Read the model definition and answer for the solid it produces. Units are mm, in the model's axes. Face numbers are marked on the shaded views. A direction names the side the tool comes from. Coordinates: 2 decimals unless noted, no trailing zeros. Order: outer loops, then holes, each group sorted by start corner. A loop starts at its lowest first (then second) coordinate and runs counter-clockwise, first axis right, second up. Notation, with made-up numbers: (36.5, 26.25) - (91.5, 26.25) arc R18 cw to (91.5, 49.25) - close; hole circle Ø4 at (66, 86). An arc over 180 degrees is marked (long way). Write item = value, one per line.
from build123d import *

# Parameters (mm, degrees)
F0_W     = 10.414
F0_H     = 140.97
F1_DEPTH = 1.27
F2_W     = 10.414
F2_H     = 1.27
F3_DEPTH = 67.564
F4_DEPTH = 67.564
F6_DEPTH = 1.27
F8_DEPTH = 1.27


with BuildPart() as f1:
    # F0 (on Top) → F1 (new body)
    with BuildSketch(Plane.XY):
        Rectangle(F0_W, F0_H)
    extrude(amount=F1_DEPTH)

    # F2 (on face) → F3 (join)
    with BuildSketch(Plane.XY.offset(1.27)):
        with Locations((0, -69.85)):
            Rectangle(F2_W, F2_H)
    extrude(amount=F3_DEPTH)

    # F2 (on face) → F4 (join)
    with BuildSketch(Plane.XY.offset(1.27)):
        with Locations((0, 69.85)):
            Rectangle(F2_W, F2_H)
    extrude(amount=F4_DEPTH)

    # F5 (on face) → F6 (join)
    with BuildSketch(Plane.YZ.offset(5.207)):
        Polygon((69.215, 1.27), (-69.215, 68.834), (-69.215, 1.27), align=None)
    extrude(amount=-F6_DEPTH)

    # F7 (on face) → F8 (join)
    with BuildSketch(Plane(origin=(-5.207, 0, 0), x_dir=(0, -1, 0), z_dir=(-1, 0, 0))):
        Polygon((69.215, 1.27), (-69.215, 68.834), (-69.215, 1.27), align=None)
    extrude(amount=-F8_DEPTH)


solid = f1.part
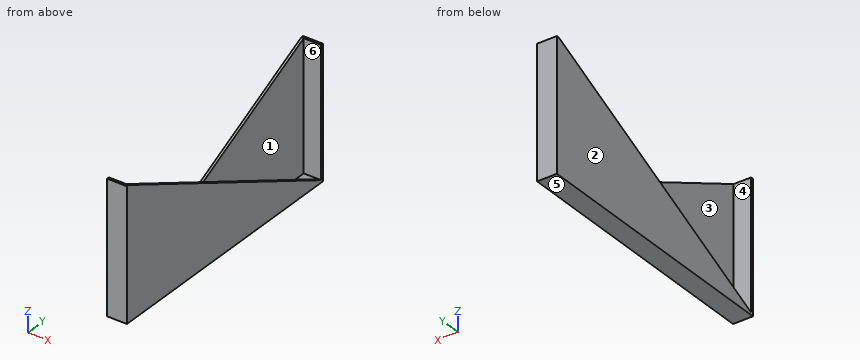
1) The part is cut by section D-D (z = 28). Determine the outline of the cut face in (x, y) (3 decimals), and give its area (3 significant figures).
Returned:
outline = (-5.207, -70.485) - (5.207, -70.485) - (5.207, 14.449) - (3.937, 14.449) - (3.937, -69.215) - (-5.207, -69.215) - close; (-5.207, -14.449) - (-3.937, -14.449) - (-3.937, 69.215) - (5.207, 69.215) - (5.207, 70.485) - (-5.207, 70.485) - close
area = 239 mm^2
2) The part is cut by section A-A (z = 48.5). Determine the outline of the cut face in (x, y) (3 decimals).
Returned:
outline = (-5.207, -70.485) - (5.207, -70.485) - (5.207, -27.553) - (3.937, -27.553) - (3.937, -69.215) - (-5.207, -69.215) - close; (-5.207, 27.553) - (-3.937, 27.553) - (-3.937, 69.215) - (5.207, 69.215) - (5.207, 70.485) - (-5.207, 70.485) - close
3) Straight lines are drawn through the part: line 1 along Y through (x, z) = (3.75, 46.5) (3 decimals); line 2 along X through (y, z) = (-4, 29); line 3 along X through (y, z) = (61, 23.5). For each, find the intervals that lie inside material, in ascending order. Write a range as from..to.
Returned:
line_1 = -70.485..-69.215, 69.215..70.485
line_2 = -5.21..-3.94, 3.94..5.21
line_3 = -5.21..-3.94
4) For the marked faces 5 and 6, determine the directions among +Z, -Z, +X, -X, +Y, -Y from which every point of the face is accessible in a straight line to the end or side of a thin tool.
Returned:
face_5 = -Z, +X, -X, +Y, -Y
face_6 = +Z, +X
5) The part is cut by section C-C (y = 18). Determine the outline of the cut face in (x, z).
Returned:
outline = (-5.21, 0) - (5.21, 0) - (5.21, 26.27) - (3.94, 26.27) - (3.94, 1.27) - (-3.94, 1.27) - (-3.94, 43.84) - (-5.21, 43.84) - close
6) Determine the mould class of the marked faces 1, 2, 3 and 4 for opening direction X: pulls with the +X half, pulls with the -X half, needs draft (parallel to the pull), parting line crosses it, or undercut.
Returned:
face_1 = undercut
face_2 = pulls with the -X half
face_3 = undercut
face_4 = needs draft
7) The part is cut by section B-B (x = -1.75). Determine the outline of the cut face in (y, z) (3 decimals), and give its area (3 significant figures).
Returned:
outline = (-70.485, 0) - (70.485, 0) - (70.485, 68.834) - (69.215, 68.834) - (69.215, 1.27) - (-69.215, 1.27) - (-69.215, 68.834) - (-70.485, 68.834) - close
area = 351 mm^2
8) A flat-ended cylindrical pin translates along its axis: pin 1 Ø2 at (x, y) = (-2.5, -19) entering from +Z. Find the tip coordinate at first contact, or state that the pin passes through.
Returned:
pin_1 = 1.27
